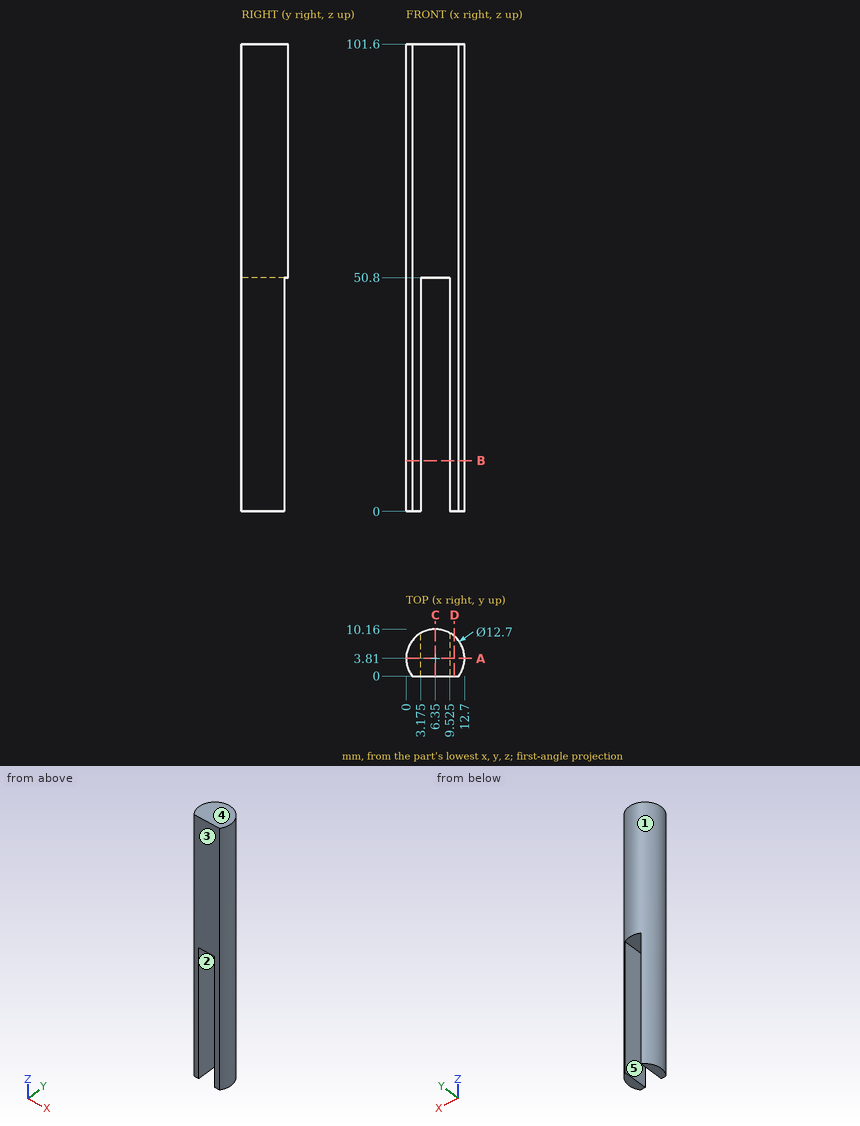
Design review of the part shown in the three views and the two pictorial views. Dimensions are in mm from the part's minimum x, y and z. A direction names the side the tool comes from. Round coordinates to 2 decimals unless told otherwise and drop trailing zeros. Order: outer loops, then holes, each group sorted by start corner. A loop starts at its lowest first (then second) coordinate and runs counter-clockwise, first axis right, second up.
Item 1: Add section A-A, the plane y = 3.81. State the section outline as (x, z) points (3 decimals).
Working result:
outline: (0, 0) - (3.175, 0) - (3.175, 50.8) - (9.525, 50.8) - (9.525, 0) - (12.7, 0) - (12.7, 101.6) - (0, 101.6) - close
Item 2: To check wall thickness, follow probe 1 along X at (y, z) = (3.5, 17) (3 decimals); probe 2 along Z at (x, y) = (6.5, 8.5); probe 3 along X at (y, z) = (8, 11) (3 decimals). State the ranges of each line that lie inside material, in increasing order.
Working result:
probe 1: x = 0.008 to 3.175, 9.525 to 12.692
probe 2: z = 50.8 to 101.6
probe 3: x = 1.579 to 3.175, 9.525 to 11.121
Item 3: Draft analysis for pull direction X (two halves, no side actions). For the marked faces 1, 2 and 3, state which applies: released by +X, released by -X, zero draft, split by the parting line, or undercut.
Working result:
face 1: split by the parting line
face 2: undercut
face 3: zero draft
Item 4: Add section C-C, the plane x = 6.35. State the section outline as (y, z) points.
Working result:
outline: (0, 50.8) - (10.16, 50.8) - (10.16, 101.6) - (0, 101.6) - close
Item 5: Add section D-D, the plane x = 10.5. State the section outline as (y, z) points.
Working result:
outline: (0, 0) - (8.62, 0) - (8.62, 101.6) - (0, 101.6) - close
Item 6: Add section B-B, the plane z = 11. State the section outline as (x, y) points (3 decimals).
Working result:
outline: (1.27, 0) - (3.175, 0) - (3.175, 9.309) arc R6.35 ccw to start; (9.525, 0) - (11.43, 0) arc R6.35 ccw to (9.525, 9.309) - close
Item 7: For pin 1 (3 mm diameter, centred on y = 4.5, z = 32, fed in from +X); pin 2 (1 mm diameter, centred on x = 4.5, z = 82.5, fed in from +Y); pin 3 (3 mm diameter, centred on x = 5.5, y = 5.5, fed in from -Z); pin 4 (1 mm diameter, centred on y = 6, z = 18, fed in from +X), all flat-tipped, find the tip position at first contact; note any pin that passes through.
Working result:
pin 1: stops at x = 12.7
pin 2: stops at y = 10.01
pin 3: stops at z = 50.8
pin 4: stops at x = 12.47
Item 8: Machinability: for the marked faces 4 and 5, which of the approach directions +Z, -Z, +X, -X, +Y, -Y give a long, thin tool a straight path to every point of the face, cutting with its end or side? Answer none if there is none.
Working result:
face 4: +Z, +X, -X, +Y, -Y
face 5: -Z, +Y, -Y
